from build123d import *

# Parameters (mm, degrees)
F0_R     = 14.2875
F0_R_2   = 10.9982
F1_DEPTH = 6.35


with BuildPart() as f1:
    # F0 (on Front) → F1 (new body)
    with BuildSketch(Plane.XZ):
        with BuildLine():
            ThreePointArc((-0.5844780805, 14.2755399766), (9.8939861955, 10.3073611275), (14.2875, 0))
            ThreePointArc((14.2875, 0), (10.1027881233, -10.1027881491), (-3.66e-08, -14.2875))
            ThreePointArc((-3.66e-08, -14.2875), (18.5132722505, -19.415379547), (31.75, -33.3375))
            ThreePointArc((31.75, -33.3375), (42.3151393195, -18.1350597083), (46.0375, 0))
            ThreePointArc((46.0375, 0), (42.3151393195, 18.1350597083), (31.75, 33.3375))
            ThreePointArc((31.75, 33.3375), (17.9746422802, 19.7492124484), (-0.5844780805, 14.2755399766))
        make_face()
        with Locations((31.75, 0)):
            Circle(F0_R, mode=Mode.SUBTRACT)
        with BuildLine():
            ThreePointArc((-3.66e-08, -14.2875), (-14.2845096816, -0.2923001993), (-0.5844780805, 14.2755399766))
            ThreePointArc((-0.5844780805, 14.2755399766), (-19.5289453165, 18.2137151613), (-34.3690170298, 30.6304109449))
            ThreePointArc((-34.3690170298, 30.6304109449), (-43.021593548, 16.3888344563), (-46.0375, 1.611e-07))
            ThreePointArc((-46.0375, 1.611e-07), (-42.3151393512, -18.1350596343), (-31.75, -33.3375))
            ThreePointArc((-31.75, -33.3375), (-18.5132722818, -19.4153795658), (-3.66e-08, -14.2875))
        make_face()
        with BuildLine():
            ThreePointArc((-17.4625, 0), (-31.7500000805, -14.2875), (-46.0375, 1.611e-07))
            ThreePointArc((-46.0375, 1.611e-07), (-31.7499999195, 14.2875), (-17.4625, 0))
        make_face(mode=Mode.SUBTRACT)
        with BuildLine():
            ThreePointArc((-3.66e-08, -14.2875), (10.1027881233, -10.1027881491), (14.2875, 0))
            ThreePointArc((14.2875, 0), (9.8939861955, 10.3073611275), (-0.5844780805, 14.2755399766))
            ThreePointArc((-0.5844780805, 14.2755399766), (-14.2845096816, -0.2923001993), (-3.66e-08, -14.2875))
        make_face()
        Circle(F0_R_2, mode=Mode.SUBTRACT)
        with Locations((31.75, 0)):
            Circle(F0_R)
        with Locations((31.75, 0)):
            Circle(F0_R_2, mode=Mode.SUBTRACT)
        with BuildLine():
            ThreePointArc((-17.4625, 0), (-31.7499999195, 14.2875), (-46.0375, 1.611e-07))
            ThreePointArc((-46.0375, 1.611e-07), (-31.7500000805, -14.2875), (-17.4625, 0))
        make_face()
        with Locations((-31.75, 0)):
            Circle(F0_R_2, mode=Mode.SUBTRACT)
    extrude(amount=F1_DEPTH)


solid = f1.part
Design review of the part built by this model. Coordinates are the model's own, in mm. Round coordinates to 2 decimals unless told otherwise and drop trailing zeros. Write each loop counter-clockwise with the first axis right and the second up, starting at its lowest first coordinate (ties: lowest second). Pieces come first, ordered by that corner, then holes. Notation, with made-up numbers: M -39,-9.75 L 3,-9.75 A17 ccw 3,3.25 Z; hole C 49,39 d3. An arc over 180 degrees is marked long. One line per item, written item: value. Start each with the question number.
1. Take a section at C-C on x = -25. State the section outline as (y, z) points.
2. Draft analysis for pull direction Z (two halves, no side actions). For faces 1 (the face through (-8.73, -3.13, -6.69)), 2 (the face through (10, -6.35, -7)), state which applies: pulls with the +Z half, pulls with the -Z half, needs draft (parallel to the pull), parting line crosses it, or undercut.
3. Take a section at B-B on z = 28.5. State the section outline as (x, y) points, then the cut area to 3 significant figures.
4. Clearance check with flat-ended pins moving along their axes: P1, Ø1.5, axis at y = -2.5, z = -3, coming from the -X side; P2, Ø3, axis at x = -26.5, y = -4, coming from the -Z side. State where each tip first meets the part, or that it passes through.
5. Take a section at D-D on z = 5.5. State the section outline as (x, y) points.
6. To check wall thickness, follow probe 1 along X at (y, z) = (-5.25, -3.5); probe 2 along X at (y, z) = (-3.5, 4); probe 3 along X at (y, z) = (-2, 19). State the ranges of each line that lie inside material, in increasing order. Write a range as from..to.
7. Take a section at A-A on y = -2.5. State how many separate pieces and enclosed holes the cut face has, then the cut area to 3 significant figures.
Computed:
1. outline: M -6.35,-24.39 L 0,-24.39 L 0,-8.68 L -6.35,-8.68 Z; M -6.35,8.68 L 0,8.68 L 0,21.42 L -6.35,21.42 Z
2. face 1: undercut
2. face 2: needs draft
3. outline: M -36.16,-6.35 L -32.71,-6.35 L -32.71,0 L -36.16,0 Z; M 28.29,-6.35 L 36.16,-6.35 L 36.16,0 L 28.29,0 Z
3. area: 71.9 mm²
4. P1: stops at x = -45.98
4. P2: stops at z = -27.67
5. outline: M -45.71,-6.35 L -41.27,-6.35 L -41.27,0 L -45.71,0 Z; M -22.23,-6.35 L -9.52,-6.35 L -9.52,0 L -22.23,0 Z; M 9.52,-6.35 L 22.23,-6.35 L 22.23,0 L 9.52,0 Z; M 41.27,-6.35 L 45.71,-6.35 L 45.71,0 L 41.27,0 Z
6. probe 1: x = -45.9..-42.18, -21.32..-10.43, 10.43..21.32, 42.18..45.9
6. probe 2: x = -45.86..-42, -21.5..-10.25, 10.25..21.5, 42..45.86
6. probe 3: x = -41.93..-21.07, 16.65..41.93
7. separate pieces: 1
7. enclosed holes: 3
7. area: 2,640 mm²
